Work out the finished part from the listing and answer in its coordinate system (mm). A direction names the side the tool comes from. Coordinates: 2 decimals unless noted, no trailing zeros. Write each loop counter-clockwise with the first axis right and the second up, starting at its lowest first coordinate (ties: lowest second). Pieces come first, ordered by that corner, then holes. Notation, with made-up numbers: (83.25, 10.5) -> (100.25, 10.5) arc R10 cw to (100.25, 20.5) -> close; hole circle Ø3 at (52, 50.25). An arc over 180 degrees is marked (long way). Write each question's results on one line, items separated by ' | '. Start each with the question number.
Solid Edge part; units mm, degrees
sketch "Sketch1" plane through (0, 0, 0) normal (0, 0, 1) x (1, 0, 0)
  arc A0 (20.5728, 14.9176) -> (4, -26.4839) centre (64, -26.4839) ccw
  line L0 (4, -60) -> (4, -26.4839)
  line L1 (-4, -60) -> (-4, -24.6779)
  arc A1 (-4, -24.6779) -> (-5.9217, -0.9662) centre (-151.25, -24.6779) ccw
  arc A2 (14.5451, 20.165) -> (-2.9494, 5.225) centre (-32.4437, 57.4753) cw
  arc A3 (4, -60) -> (-4, -60) centre (0, -60) cw
  arc A4 (-5.9217, -0.9662) -> (-2.9494, 5.225) centre (0, 0) cw
  arc A5 (14.5451, 20.165) -> (20.5728, 14.9176) centre (17.6777, 17.6777) cw
extrude "Protrusion1" add sketch "Sketch1" along normal blind 6
sketch "Sketch2" plane through (7.8388, -21.1612, 6) normal (0, 0, 1) x (0, 1, 0)
  circle A0 centre (21.1612, 7.8388) radius 1.625
  circle A1 centre (38.8388, -9.8388) radius 1.625
extrude "VaciadoExtruido_1" cut sketch "Sketch2" against normal blind 5
sketch "Sketch3" plane through (7.8388, -21.1612, 6) normal (0, 0, 1) x (0, 1, 0)
  circle A0 centre (-38.8388, 7.8388) radius 2
  circle A1 centre (-8.8388, 7.8388) radius 2
extrude "Cutout1" cut sketch "Sketch3" against normal through all
chamfer "Chaflán_1" distance 0.5 angle 45 18 edges at (4, -43.2419, 6) (0, -64, 6) (-4, -42.339, 6) (-4.4812, -12.7832, 6) (-5.409, 2.5967, 6) (6.5206, 11.8487, 6) (20.3041, 20.6946, 6) (8.2971, -4.1862, 6) (4, -43.2419, 0) (0, -64, 0) (-4, -42.339, 0) (-4.4812, -12.7832, 0) (-5.409, 2.5967, 0) (6.5206, 11.8487, 0) (20.3041, 20.6946, 0) (8.2971, -4.1862, 0) (0, -1.625, 6) (17.6777, 16.0527, 6)
1. Given pin 1 Ø2.5 at (x, y) = (17, 18) entering from +Z; pin 2 Ø1.5 at (y, z) = (-18.5, 2.5) entering from -X; pin 3 Ø2.5 at (y, z) = (-44, 3) entering from +X, each flat-ended and moving along its own axis, determine where each tip first touches the part or whether it passes through.
2. For faces 1 (the face through (-4, -43, 3)), 2 (the face through (4, -43, 3)), 3 (the face through (18, 18, 1)), 4 (the face through (0.08, -63.64, 5.86)), determine the directions among +Z, -Z, +X, -X, +Y, -Y from which every point of the face is accessible in a straight line to the end or side of a thin tool.
3. Find section C-C on y = -41.5. Give the vertices of the cut face in (x, z).
4. Determine the mould class of faces 5 (the face through (8.18, -4.48, 2.96)), 6 (the face through (6.64, 11.95, 2.96)), 7 (the face through (3, -15, 6)), 8 (the face through (19.12, 18.43, 3.28)) for opening direction Y: pulls with the +Y half, pulls with the -Y half, needs draft (parallel to the pull), parting line crosses it, or undercut.
5. Find the intervals of material crossed by L1, parallel to Y at x = 0, z = 3.75 (3 decimals); L2, parallel to X at y = -30, z = 3.75; L3, parallel to X at y = -33.5, z = 1.75, in increasing order.
6. Find section A-A on y = -30. Give the vertices of the cut face in (x, z).
7. Find section D-D on x = 0. Give the number of separate pieces and of enclosed holes in the cut face, and give its area (3 significant figures).
8. Find section B-B on z = 2. Give the vertices of the cut face in (x, y) (3 decimals), and give its area (3 significant figures).
Ans:
1) pin 1: stops at z = 5.88 | pin 2: stops at x = -4.16 | pin 3: stops at x = 4
2) face 1: +Z, -Z, -X, -Y | face 2: +Z, -Z, +X, -Y | face 3: +Z | face 4: +Z, -Y
3) outline: (-4, 0.5) -> (-3.5, 0) -> (3.5, 0) -> (4, 0.5) -> (4, 5.5) -> (3.5, 6) -> (-3.5, 6) -> (-4, 5.5) -> close
4) face 5: pulls with the -Y half | face 6: pulls with the +Y half | face 7: needs draft | face 8: undercut
5) L1: y = -64 to -62, -58 to -32, -28 to -1.625, 1.625 to 7.003 | L2: x = -4 to -2, 2 to 4 | L3: x = -4 to 4
6) outline: (-4, 0.5) -> (-3.5, 0) -> (-2, 0) -> (-2, 6) -> (-3.5, 6) -> (-4, 5.5) -> close; (2, 0) -> (3.5, 0) -> (4, 0.5) -> (4, 5.5) -> (3.5, 6) -> (2, 6) -> close
7) separate pieces: 3 | enclosed holes: 0 | area: 361 mm²
8) outline: (-5.922, -0.966) arc R147.25 cw to (-4, -24.678) -> (-4, -60) arc R4 ccw to (4, -60) -> (4, -26.484) arc R60 cw to (20.573, 14.918) arc R4 ccw (long way) to (14.545, 20.165) arc R60 cw to (-2.949, 5.225) arc R6 ccw to start; hole circle Ø4 at (0, -60); hole circle Ø4 at (0, -30); hole circle Ø3.25 at (0, 0); hole circle Ø3.25 at (17.678, 17.678) | area: 796 mm²
